```python
from build123d import *

# Parameters (mm, degrees)
SKETCH1_W           = 92.09999995
SKETCH1_H           = 82
BOSS_EXTRUDE3_DEPTH = 6.35
SKETCH2_W           = 12.7
SKETCH2_H           = 12.7
BOSS_EXTRUDE4_DEPTH = 59.8


with BuildPart() as part:
    # Sketch1 → Boss-Extrude3 (new body)
    with BuildSketch(Plane(origin=(0, 0, 0), x_dir=(1, 0, 0), z_dir=(0, 1, 0))):
        Rectangle(SKETCH1_W, SKETCH1_H)
    extrude(amount=BOSS_EXTRUDE3_DEPTH)

    # Sketch2 → Boss-Extrude4 (add)
    with BuildSketch(Plane(origin=(0, 6.35, 0), x_dir=(1, 0, 0), z_dir=(0, 1, 0))):
        with Locations((-39.699999975, 34.65)):
            Rectangle(SKETCH2_W, SKETCH2_H)
        with Locations((39.699999975, 34.65)):
            Rectangle(SKETCH2_W, SKETCH2_H)
        with Locations((39.699999975, -34.65)):
            Rectangle(SKETCH2_W, SKETCH2_H)
        with Locations((-39.699999975, -34.65)):
            Rectangle(SKETCH2_W, SKETCH2_H)
    extrude(amount=BOSS_EXTRUDE4_DEPTH)


solid = part.part
```
Check sheet for the modelled part. Datum: model origin and axes. Units: mm. A direction names the side the tool comes from. Give positions to 0.01 mm unless a question says otherwise; leave off trailing zeros. Order: outer loops, then holes, each group sorted by start corner. A loop starts at its lowest first (then second) coordinate and runs counter-clockwise, first axis right, second up. Notation, with made-up numbers: M 0.5,26.5 L 16.5,26.5 A31 ccw 16.5,55.5 Z; hole C 53.5,85 d6. An arc over 180 degrees is marked long. Answer in a Markdown table with one row per item.
1) Access from +Z, -Z, +X, -X, +Y, -Y to the whole of each face (thin tool, end or side, straight path). Record for faces 1 (the flat face through (-40, 36, 28.3)), 2 (the flat face through (-33.35, 36, -35)), 3 (the flat face through (0, 1, 41)).
Filled sheet:
| item | result |
|---|---|
| face 1 | +X, -X, +Y |
| face 2 | +Z, -Z, +Y |
| face 3 | +Z, +X, -X, +Y, -Y |
2) Gauge pin test, flat end, axial feed: P1, Ø10, axis at x = 35.5, z = -6, coming from the +Y side. Record the tip position at first contact, or that the pin passes through.
Filled sheet:
| item | result |
|---|---|
| P1 | stops at y = 6.35 |
3) Release check for a two-part mould opening along X. For faces 4 (the flat face through (33.35, 36, 35)), 5 (the flat face through (-46.05, 1, 0)), 6 (the flat face through (-33.35, 36, 35)), 7 (the flat face through (40, 36, 28.3)) record: +X half, -X half, draft (parallel to the pull), parting line (faces both ways), or undercut.
Filled sheet:
| item | result |
|---|---|
| face 4 | undercut |
| face 5 | -X half |
| face 6 | undercut |
| face 7 | draft |
4) Cross-section at B-B, the plane z = -30. Enter the section's corners in (x, y).
Filled sheet:
| item | result |
|---|---|
| outline | M -46.05,0 L 46.05,0 L 46.05,66.15 L 33.35,66.15 L 33.35,6.35 L -33.35,6.35 L -33.35,66.15 L -46.05,66.15 Z |
5) Thickness scan on L1, parallel to Z at x = -37.5, y = 50.5; L2, parallel to X at y = 55, z = 34; L3, parallel to Y at x = 25.5, z = -17.5. Record the ranges inside material, lowest first. Write a range as [from, to].
Filled sheet:
| item | result |
|---|---|
| L1 | z = [-41, -28.3], [28.3, 41] |
| L2 | x = [-46.05, -33.35], [33.35, 46.05] |
| L3 | y = [0, 6.35] |
6) Cross-section at A-A, the plane y = 8. Enter the section's corners in (x, z).
Filled sheet:
| item | result |
|---|---|
| outline | M -46.05,-41 L -33.35,-41 L -33.35,-28.3 L -46.05,-28.3 Z; M -46.05,28.3 L -33.35,28.3 L -33.35,41 L -46.05,41 Z; M 33.35,-41 L 46.05,-41 L 46.05,-28.3 L 33.35,-28.3 Z; M 33.35,28.3 L 46.05,28.3 L 46.05,41 L 33.35,41 Z |
7) Cross-section at D-D, the plane z = 24. Enter the section's corners in (x, y), plus the area to 3 significant figures.
Filled sheet:
| item | result |
|---|---|
| outline | M -46.05,0 L 46.05,0 L 46.05,6.35 L -46.05,6.35 Z |
| area | 585 mm2 |
8) Cross-section at C-C, the plane x = 8.5. Enter the section's corners in (y, z), plus the area to 3 significant figures.
Filled sheet:
| item | result |
|---|---|
| outline | M 0,-41 L 6.35,-41 L 6.35,41 L 0,41 Z |
| area | 521 mm2 |
